from build123d import *

# Parameters (mm, degrees)
HEX_EXTRUDE_DEPTH        = 6.35
SKETCH4_OUTSIDE_W        = 77.352
SKETCH4_OUTSIDE_H        = 79.072
SKETCH4_OUTSIDE_R        = 5.55625
HEX_CUT1_DEPTH           = 17.278326973
HEX_CUT1_DRAFT           = -60
SKETCH5_OUTSIDE_W        = 60.292
SKETCH5_OUTSIDE_H        = 62.012
SKETCH5_OUTSIDE_R        = 5.55625
HEX_CUT2_DEPTH           = 12.353215031
HEX_CUT2_DRAFT           = -60
SKETCH6_R                = 1.5875
ECCENTRIC_HOLE_CUT_DEPTH = 17.278326973
FILLET_2_R               = 0.508


with BuildPart() as part:
    # Sketch2 → Body Revolve (revolve)
    with BuildSketch(Plane(origin=(0, 0, 0), x_dir=(0, 0, -1), z_dir=(1, 0, 0)), mode=Mode.PRIVATE) as body_revolve_sk:
        Polygon((-6.9453125, 0), (6.9453125, 0), (6.9453125, 5.55625), (0.5953125, 5.55625), (0.5953125, 2.38125), (-6.9453125, 2.38125), align=None)
    revolve(body_revolve_sk.sketch.rotate(Axis((0, 0, 6.9453125), (0, 0, -1)), 90), axis=Axis((0, 0, 6.9453125), (0, 0, -1)))

    # Sketch3 → Hex Extrude (add)
    with BuildSketch(Plane(origin=(0, 0, -6.9453125), x_dir=(-1, 0, 0), z_dir=(0, 0, -1))):
        Polygon((0, 6.415804866), (-5.55625, 3.207902433), (-5.55625, -3.207902433), (0, -6.415804866), (5.55625, -3.207902433), (5.55625, 3.207902433), align=None)
    extrude(amount=-HEX_EXTRUDE_DEPTH)


with BuildPart() as hex_cut1_tool:
    # Sketch4 outside → Hex Cut1 (with draft: the straight prism first)
    with BuildSketch(Plane(origin=(0, 0, -6.9453125), x_dir=(-1, 0, 0), z_dir=(0, 0, -1))):
        Rectangle(SKETCH4_OUTSIDE_W, SKETCH4_OUTSIDE_H)
        Circle(SKETCH4_OUTSIDE_R, mode=Mode.SUBTRACT)
    extrude(amount=-HEX_CUT1_DEPTH)
    # Hex Cut1: the draft: its side faces are tilted about the plane it starts from
    hex_cut1_sides = [hex_cut1_tool.faces().sort_by_distance(p)[0] for p in [
        (0, -39.536, 1.693850986),
        (-38.676, 0, 1.693850986),
        (0, 39.536, 1.693850986),
        (38.676, 0, 1.693850986),
        (5.55625, 0, 1.693850986),
    ]]
    draft(hex_cut1_sides, Plane(origin=(0, 0, -6.9453125), x_dir=(-1, 0, 0), z_dir=(0, 0, -1)), HEX_CUT1_DRAFT)


with BuildPart() as part_1:
    add(part.part)

    # Hex Cut1: cut by hex_cut1_tool
    add(hex_cut1_tool.part, mode=Mode.SUBTRACT)


with BuildPart() as hex_cut2_tool:
    # Sketch5 outside → Hex Cut2 (with draft: the straight prism first)
    with BuildSketch(Plane.XY.offset(-0.5953125)):
        Rectangle(SKETCH5_OUTSIDE_W, SKETCH5_OUTSIDE_H)
        Circle(SKETCH5_OUTSIDE_R, mode=Mode.SUBTRACT)
    extrude(amount=-HEX_CUT2_DEPTH)
    # Hex Cut2: the draft: its side faces are tilted about the plane it starts from
    hex_cut2_sides = [hex_cut2_tool.faces().sort_by_distance(p)[0] for p in [
        (0, -31.006, -6.771920015),
        (30.146, 0, -6.771920015),
        (0, 31.006, -6.771920015),
        (-30.146, 0, -6.771920015),
        (-5.55625, 0, -6.771920015),
    ]]
    draft(hex_cut2_sides, Plane.XY.offset(-0.5953125), HEX_CUT2_DRAFT)


with BuildPart() as part_2:
    add(part_1.part)

    # Hex Cut2: cut by hex_cut2_tool
    add(hex_cut2_tool.part, mode=Mode.SUBTRACT)

    # Sketch6 → Eccentric Hole Cut (cut, through all)
    with BuildSketch(Plane.XY.offset(6.9453125)):
        with Locations((0, -0.3048)):
            Circle(SKETCH6_R)
    extrude(amount=-ECCENTRIC_HOLE_CUT_DEPTH, mode=Mode.SUBTRACT)

    # Fillet 2
    fillet_2_edges = [part_2.edges().sort_by_distance(p)[0] for p in [
        (-2.38125, 0, 6.9453125),
        (-2.38125, 0, -0.5953125),
    ]]
    fillet(fillet_2_edges, radius=FILLET_2_R)

    # Chamfer 2: read off the stored shape, not the designer's step
    # Chamfer 2 outline → Chamfer 2 (revolve, cut)
    with BuildSketch(Plane.XZ.offset(0.3048)):
        Polygon((1.5875, 6.945313993), (1.5875, 6.746875), (1.785938993, 6.945313993), align=None)
        Polygon((1.7859375, -6.9453125), (1.5875, -6.746875), (1.5875, -6.9453125), align=None)
    revolve(axis=Axis((0, -0.3048, 0), (0, 0, 1)), mode=Mode.SUBTRACT)


solid = part_2.part
Could you check a few things on this model? Use its own coordinates, in mm. Give positions to 0.01 mm unless a question says otherwise; leave off trailing zeros. Loops run counter-clockwise (first coordinate to the right, second up) from the corner with the lowest first, then second, coordinate; pieces in that order, holes last. Notation, with made-up numbers: (55, 50) -> (74, 50) arc R23 cw to (74, 68) -> close; hole circle Ø5 at (34.25, 55). An arc over 180 degrees is marked (long way). Return JSON: item names as keys, results as strings.
Item 1: If we section it at A-A on z = 3.5: List the corners of the cut face in (x, y) for me (1 decimal), plus the area to 3 significant figures.
Geometry results:
{"outline": "circle Ø4.8 at (0, 0); hole circle Ø3.2 at (0, -0.3)", "area": "9.90 mm²"}
Item 2: I need wall thicknesses on L1, parallel to Y at x = 0, z = 1.25; L2, parallel to Z at x = 4.75, y = 0.5; L3, parallel to X at y = 5.5, z = -5. Which ranges of each line are inside material? Lowest first, please. Write a range as from..to.
Geometry results:
{"L1": "y = -2.38..-1.89, 1.28..2.38", "L2": "z = -6.95..-0.6", "L3": "x = -1.59..1.59"}
Item 3: I'm going to push flat-ended pins straight in: pin 1 (4 mm diameter, centred on x = -2, z = 2, fed in from +Y); pin 2 (2 mm diameter, centred on y = -2.5, z = 4.5, fed in from -X); pin 3 (5 mm diameter, centred on x = -3.5, z = 4.5, fed in from -Y). Where does each tip first touch, or does it pass through?
Geometry results:
{"pin 1": "stops at y = 2.38", "pin 2": "stops at x = -1.85", "pin 3": "stops at y = -2.16"}
Item 4: We'd pull the mould along Y, two halves only. Please class faces 1 (the flat face through (-5.556, 0, -4)), 2 (the conical face through (4.98, -2.89, -0.71)), 3 (the cylindrical face through (1.514, 0.172, 0.094)): +Y half, -Y half, draft (parallel to the pull), parting line (faces both ways), or undercut.
Geometry results:
{"face 1": "draft", "face 2": "-Y half", "face 3": "undercut"}
